Geometry: final body of the model. Coordinates: model frame, mm. A direction names the side the tool comes from. Coordinates: 2 decimals unless noted, no trailing zeros. Order: outer loops, then holes, each group sorted by start corner. A loop starts at its lowest first (then second) coordinate and runs counter-clockwise, first axis right, second up. Notation, with made-up numbers: (3.5, 55) - (21.5, 55) arc R34 cw to (21.5, 88) - close; hole circle Ø7 at (29.5, -4). An arc over 180 degrees is marked (long way). Use a Markdown table: item, result. Add a question column.
```python
from build123d import *

# Parameters (mm, degrees)
F1_DEPTH      = 20
F1_DEPTH_BACK = 30
F2_DEPTH      = 10


with BuildPart() as f1:
    # F0 (on Front) → F1 (new body, two sides)
    with BuildSketch(Plane.XZ) as f1_sk:
        Polygon((2.03516, -1.175), (2.03516, 1.175), (0, 2.35), (-2.03516, 1.175), (-2.03516, -1.175), (0, -2.35), align=None)
    extrude(amount=F1_DEPTH)
    extrude(f1_sk.sketch, amount=-F1_DEPTH_BACK)

    # F0 (on Front) → F2 (join)
    with BuildSketch(Plane.XZ):
        with BuildLine():
            Line((-2.03516, 1.175), (0, 2.35))
            ThreePointArc((0, 2.35), (-1.175, 2.03516), (-2.03516, 1.175))
        make_face()
        with BuildLine():
            Line((0, 2.35), (2.03516, 1.175))
            ThreePointArc((2.03516, 1.175), (1.175, 2.03516), (0, 2.35))
        make_face()
        with BuildLine():
            ThreePointArc((2.03516, -1.175), (2.269926, -0.608225), (2.35, 0))
            ThreePointArc((2.35, 0), (2.269926, 0.608225), (2.03516, 1.175))
            Line((2.03516, 1.175), (2.03516, -1.175))
        make_face()
        with BuildLine():
            ThreePointArc((0, -2.35), (1.175, -2.03516), (2.03516, -1.175))
            Line((2.03516, -1.175), (0, -2.35))
        make_face()
        Polygon((2.03516, -1.175), (2.03516, 1.175), (0, 2.35), (-2.03516, 1.175), (-2.03516, -1.175), (0, -2.35), align=None)
        with BuildLine():
            Line((-2.03516, -1.175), (-2.03516, 1.175))
            ThreePointArc((-2.03516, 1.175), (-2.35, 0), (-2.03516, -1.175))
        make_face()
        with BuildLine():
            ThreePointArc((-2.03516, -1.175), (-1.175, -2.03516), (0, -2.35))
            Line((0, -2.35), (-2.03516, -1.175))
        make_face()
    extrude(amount=-F2_DEPTH)


solid = f1.part
```
1) Pin query (flat end, axial travel): pin 1 (1.5 mm diameter, centred on y = -3.5, z = 1.5, fed in from -X); pin 2 (1 mm diameter, centred on x = 1, y = -13.5, fed in from +Z); pin 3 (1.5 mm diameter, centred on x = 0.5, y = -2.5, fed in from -Z). Return the tip coordinate at first contact, or that it passes through.
2) Set-up query: faces 1 (the face through (2.035, 20, 0)), 2 (the face through (-1.1, 10, -1.9)), 3 (the face through (-1.003, -10.14, 1.771)). Return all of +Z, -Z, +X, -X, +Y, -Y with unobstructed straight access to the full face (end or side cutting, diameter ignored); none if empty.
3) Section B-B (z = 0.5). Return loops of the section in (x, y), then the cut area to 3 significant figures.
4) Ray query, line 1 along Y through (x, z) = (-0.85, 2); line 2 along X through (y, z) = (19.5, 0.3); line 3 along Z through (x, y) = (0.1, 4). Return the intervals inside material, ascending.
5) Section C-C (x = 0.7). Return loops of the section in (y, z).
6) Section A-A (y = 6.5). Return loops of the section in (x, z) (3 decimals), then the cut area to 3 significant figures.
7) Section D-D (y = -0.5). Return loops of the section in (x, z) (3 decimals).
Values follow:
| question | item | result |
|---|---|---|
| 1 | pin 1 | stops at x = -2.04 |
| 1 | pin 2 | stops at z = 2.06 |
| 1 | pin 3 | stops at z = -2.35 |
| 2 | face 1 | +Z, -Z, +X, +Y |
| 2 | face 2 | -Z, -X, +Y |
| 2 | face 3 | +Z, -X, -Y |
| 3 | outline | (-2.3, 0) - (-2.04, 0) - (-2.04, -20) - (2.04, -20) - (2.04, 0) - (2.3, 0) - (2.3, 10) - (2.04, 10) - (2.04, 30) - (-2.04, 30) - (-2.04, 10) - (-2.3, 10) - close |
| 3 | area | 209 mm² |
| 4 | line 1 | y = 0 to 10 |
| 4 | line 2 | x = -2.04 to 2.04 |
| 4 | line 3 | z = -2.35 to 2.35 |
| 5 | outline | (-20, -1.95) - (0, -1.95) - (0, -2.24) - (10, -2.24) - (10, -1.95) - (30, -1.95) - (30, 1.95) - (10, 1.95) - (10, 2.24) - (0, 2.24) - (0, 1.95) - (-20, 1.95) - close |
| 6 | outline | (-2.035, -1.175) arc R2.35 ccw to (0, -2.35) arc R2.35 ccw to (2.035, -1.175) arc R2.35 ccw to (2.35, 0) arc R2.35 ccw to (2.035, 1.175) arc R2.35 ccw to (0, 2.35) arc R2.35 ccw to (-2.035, 1.175) arc R2.35 ccw to start |
| 6 | area | 17.3 mm² |
| 7 | outline | (-2.035, -1.175) - (0, -2.35) - (2.035, -1.175) - (2.035, 1.175) - (0, 2.35) - (-2.035, 1.175) - close |
